The listing builds one solid part. Answer for the finished solid, in the listing's coordinates (mm). Round coordinates to 2 decimals unless told otherwise and drop trailing zeros. Order: outer loops, then holes, each group sorted by start corner. A loop starts at its lowest first (then second) coordinate and runs counter-clockwise, first axis right, second up. Notation, with made-up numbers: (-7, 53) - (23, 53) arc R25 cw to (23, 80) - close; hole circle Ø11 at (62, -28.75). An arc over 180 degrees is marked (long way). One line per item, written item: value. Start each with the question number.
1. Section C-C, the plane y = -20 is taken. Give the vertices of the cut face in (x, z), then the cut area to 3 significant figures.
2. Straight lines are drawn through the part: line 1 (Y direction, x = 0, z = 0.5); line 2 (Y direction, x = 2, z = 1.05); line 3 (X direction, y = -16.5, z = 0.7). For each, find the intervals that lie inside material, in ascending order.
3. A flat-ended cylindrical pin translates along its axis: P1, Ø7, axis at x = 0, y = 20, coming from the +Z side. Find the tip coordinate at first contact, or state that the pin passes through.
4. Section A-A, the plane x = 0 is taken. Give the vertices of the cut face in (y, z), then the cut area to 3 significant figures.
5. Section B-B, the plane z = 1.5 is taken. Give the vertices of the cut face in (x, y).
from build123d import *

# Parameters (mm, degrees)
SKETCH1_W           = 40
SKETCH1_H           = 80
BOSS_EXTRUDE1_DEPTH = 2
SKETCH2_R           = 4.25
CUT_EXTRUDE1_DEPTH  = 2
FILLET1_R           = 2.5


with BuildPart() as part:
    # Sketch1 → Boss-Extrude1 (new body)
    with BuildSketch(Plane.XY):
        Rectangle(SKETCH1_W, SKETCH1_H)
    extrude(amount=BOSS_EXTRUDE1_DEPTH)

    # Sketch2 → Cut-Extrude1 (cut)
    with BuildSketch(Plane.XY.offset(2)):
        with Locations((0, 20)):
            Circle(SKETCH2_R)
        with Locations((0, -20)):
            Circle(SKETCH2_R)
    extrude(amount=-CUT_EXTRUDE1_DEPTH, mode=Mode.SUBTRACT)

    # Fillet1
    fillet1_edges = [part.edges().sort_by_distance(p)[0] for p in [
        (-20, 40, 1),
        (20, 40, 1),
        (20, -40, 1),
        (-20, -40, 1),
    ]]
    fillet(fillet1_edges, radius=FILLET1_R)


solid = part.part
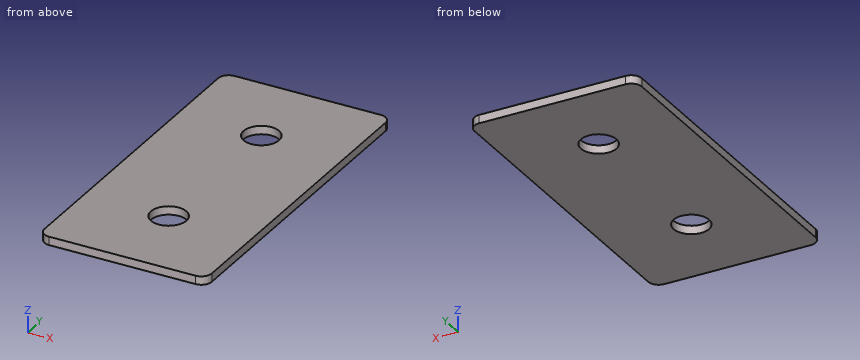
Answer list:
1. outline: (-20, 0) - (-4.25, 0) - (-4.25, 2) - (-20, 2) - close; (4.25, 0) - (20, 0) - (20, 2) - (4.25, 2) - close
1. area: 63.0 mm²
2. line 1: y = -40 to -24.25, -15.75 to 15.75, 24.25 to 40
2. line 2: y = -40 to -23.75, -16.25 to 16.25, 23.75 to 40
2. line 3: x = -20 to -2.41, 2.41 to 20
3. P1: passes through
4. outline: (-40, 0) - (-24.25, 0) - (-24.25, 2) - (-40, 2) - close; (-15.75, 0) - (15.75, 0) - (15.75, 2) - (-15.75, 2) - close; (24.25, 0) - (40, 0) - (40, 2) - (24.25, 2) - close
4. area: 126 mm²
5. outline: (-20, -37.5) arc R2.5 ccw to (-17.5, -40) - (17.5, -40) arc R2.5 ccw to (20, -37.5) - (20, 37.5) arc R2.5 ccw to (17.5, 40) - (-17.5, 40) arc R2.5 ccw to (-20, 37.5) - close; hole circle Ø8.5 at (0, -20); hole circle Ø8.5 at (0, 20)
